```python
from build123d import *

# Parameters (mm, degrees)
F1_DEPTH = 5.08


with BuildPart() as f1:
    # F0 (on Front) → F1 (new body)
    with BuildSketch(Plane.XZ):
        with BuildLine():
            add(Edge.make_bspline(
                [(-88.697367137, -151.6268995181), (-88.8096869402, -151.4451622066), (-75.5090993087, -97.1505766968), (-75.2492718061, -96.7301671852)],
                knots=[0, 0, 0, 0, 1, 1, 1, 1], degree=3))
            add(Edge.make_bspline(
                [(-81.2252771404, -151.7485828201), (-85.2727205926, -151.7823095151), (-88.6351599598, -151.727558088), (-88.697367137, -151.6268995181)],
                knots=[0, 0, 0, 0, 1, 1, 1, 1], degree=3))
            Line((-81.2252771404, -151.7485828201), (-73.8662922876, -151.6872587675))
            Line((-73.8662922876, -151.6872587675), (-70.8277989917, -141.6973681422))
            add(Edge.make_bspline(
                [(-67.6823091824, -131.3943521191), (-67.7411591055, -131.5665717782), (-69.1566280625, -136.202929372), (-70.8277989917, -141.6973681422)],
                knots=[0, 0, 0, 0, 1, 1, 1, 1], degree=3))
            add(Edge.make_bspline(
                [(-64.7710364528, -141.3842427444), (-66.3133869912, -135.7175812475), (-67.6234592594, -131.2221309262), (-67.6823091824, -131.3943521191)],
                knots=[0, 0, 0, 0, 1, 1, 1, 1], degree=3))
            Line((-64.7710364528, -141.3842427444), (-61.9667602367, -151.6872587675))
            Line((-61.9667602367, -151.6872587675), (-54.7617960796, -151.7486058281))
            add(Edge.make_bspline(
                [(-47.327106009, -151.5162830756), (-47.50533383, -151.7441177296), (-49.1720212624, -151.796198692), (-54.7617960796, -151.7486058281)],
                knots=[0, 0, 0, 0, 1, 1, 1, 1], degree=3))
            add(Edge.make_bspline(
                [(-44.3397073984, -141.4129659612), (-45.8564269984, -146.8082708266), (-47.2007536122, -151.3547652154), (-47.327106009, -151.5162830756)],
                knots=[0, 0, 0, 0, 1, 1, 1, 1], degree=3))
            add(Edge.make_bspline(
                [(-41.434975083, -131.8877223747), (-41.5158590234, -131.7313015586), (-42.8229893322, -136.0176626297), (-44.3397073984, -141.4129659612)],
                knots=[0, 0, 0, 0, 1, 1, 1, 1], degree=3))
            add(Edge.make_bspline(
                [(-38.4365004097, -141.6973681422), (-40.0047779231, -136.4584856268), (-41.3540942103, -132.0441447246), (-41.434975083, -131.8877223747)],
                knots=[0, 0, 0, 0, 1, 1, 1, 1], degree=3))
            add(Edge.make_bspline(
                [(-35.35325344, -151.5148749846), (-35.4807623735, -151.3541301939), (-36.8682228963, -146.9362537254), (-38.4365004097, -141.6973681422)],
                knots=[0, 0, 0, 0, 1, 1, 1, 1], degree=3))
            add(Edge.make_bspline(
                [(-21.618593749, -151.747197737), (-32.2466686649, -151.7943779904), (-35.1707783378, -151.744881596), (-35.35325344, -151.5148749846)],
                knots=[0, 0, 0, 0, 1, 1, 1, 1], degree=3))
            Line((-21.618593749, -151.747197737), (-8.1157690404, -151.6872587675))
            Line((-8.1157690404, -151.6872587675), (-8.0551122205, -142.1039337259))
            Line((-8.0551122205, -142.1039337259), (-7.994452333, -132.5206102182))
            Line((-7.994452333, -132.5206102182), (0.0155073543, -132.5206102182))
            Line((0.0155073543, -132.5206102182), (8.0254655077, -132.5206102182))
            Line((8.0254655077, -132.5206102182), (8.0861545387, -141.9877738836))
            Line((8.0861545387, -141.9877738836), (8.1468328327, -151.4549360151))
            Line((8.1468328327, -151.4549360151), (16.8305932312, -151.5710973913))
            add(Edge.make_bspline(
                [(25.602503504, -151.4549360151), (25.5448131854, -151.6069745696), (22.5134799865, -151.6471159016), (16.8305932312, -151.5710973913)],
                knots=[0, 0, 0, 0, 1, 1, 1, 1], degree=3))
            add(Edge.make_bspline(
                [(25.6308616602, -124.1569819276), (25.6637462615, -139.0430796988), (25.6509768084, -151.3271586547), (25.602503504, -151.4549360151)],
                knots=[0, 0, 0, 0, 1, 1, 1, 1], degree=3))
            Line((25.6308616602, -124.1569819276), (25.5710607389, -97.0913505925))
            Line((25.5710607389, -97.0913505925), (16.8589513874, -97.0913505925))
            Line((16.8589513874, -97.0913505925), (8.1468328327, -97.0913505925))
            Line((8.1468328327, -97.0913505925), (8.0863155949, -107.25548194))
            Line((8.0863155949, -107.25548194), (8.0257891539, -117.4196144379))
            Line((8.0257891539, -117.4196144379), (0.0155349639, -117.4196144379))
            Line((0.0155349639, -117.4196144379), (-7.9947238277, -117.4196144379))
            Line((-7.9947238277, -117.4196144379), (-8.055247201, -107.25548194))
            Line((-8.055247201, -107.25548194), (-8.1157690404, -97.0913505925))
            Line((-8.1157690404, -97.0913505925), (-16.0147518261, -97.0913505925))
            Line((-16.0147518261, -97.0913505925), (-23.9137330779, -97.0913505925))
            Line((-23.9137330779, -97.0913505925), (-24.029895988, -118.8869035998))
            Line((-24.029895988, -118.8869035998), (-24.1460573642, -140.682456607))
            Line((-24.1460573642, -140.682456607), (-29.34602871, -119.003064976))
            add(Edge.make_bspline(
                [(-34.7574514629, -96.9138580697), (-34.6411535724, -97.1392555987), (-32.206013487, -107.0794001925), (-29.34602871, -119.003064976)],
                knots=[0, 0, 0, 0, 1, 1, 1, 1], degree=3))
            add(Edge.make_bspline(
                [(-42.3147712321, -96.5653737493), (-35.4953141815, -96.5084380938), (-34.9537513196, -96.5334106193), (-34.7574514629, -96.9138580697)],
                knots=[0, 0, 0, 0, 1, 1, 1, 1], degree=3))
            Line((-42.3147712321, -96.5653737493), (-49.6606411279, -96.6267045125))
            Line((-49.6606411279, -96.6267045125), (-52.2309748268, -106.6762014496))
            add(Edge.make_bspline(
                [(-54.9470536187, -116.3176067958), (-54.8637032182, -116.5509909851), (-53.7009344533, -112.4234481661), (-52.2309748268, -106.6762014496)],
                knots=[0, 0, 0, 0, 1, 1, 1, 1], degree=3))
            add(Edge.make_bspline(
                [(-57.7247095515, -106.5004324194), (-56.2771582062, -111.6754283637), (-55.0272151072, -116.0931558553), (-54.9470536187, -116.3176067958)],
                knots=[0, 0, 0, 0, 1, 1, 1, 1], degree=3))
            add(Edge.make_bspline(
                [(-60.5752196243, -96.8009467685), (-60.4549888956, -96.9606688526), (-59.172257829, -101.3254374338), (-57.7247095515, -106.5004324194)],
                knots=[0, 0, 0, 0, 1, 1, 1, 1], degree=3))
            add(Edge.make_bspline(
                [(-75.2492718061, -96.7301671852), (-75.0293705104, -96.3743622869), (-60.8448337816, -96.4427814387), (-60.5752196243, -96.8009467685)],
                knots=[0, 0, 0, 0, 1, 1, 1, 1], degree=3))
        make_face()
        with BuildLine():
            add(Edge.make_bspline(
                [(-71.5440418374, -137.8059582044), (-69.5220890449, -131.1295757823), (-67.8197054306, -125.5795634317), (-67.7609690139, -125.4725960617)],
                knots=[0, 0, 0, 0, 1, 1, 1, 1], degree=3))
            Line((-71.5440418374, -137.8059582044), (-75.2203236858, -149.9448365905))
            Line((-75.2203236858, -149.9448365905), (-80.8996503329, -149.9448365905))
            add(Edge.make_bspline(
                [(-86.4738924333, -149.5382710068), (-86.5718489025, -149.9172545717), (-86.1936823142, -149.9448365905), (-80.8996503329, -149.9448365905)],
                knots=[0, 0, 0, 0, 1, 1, 1, 1], degree=3))
            add(Edge.make_bspline(
                [(-80.122365283, -123.7504163439), (-83.5579088109, -137.7101251841), (-86.4160974282, -149.3146590921), (-86.4738924333, -149.5382710068)],
                knots=[0, 0, 0, 0, 1, 1, 1, 1], degree=3))
            Line((-80.122365283, -123.7504163439), (-73.8759219124, -98.369127073))
            Line((-73.8759219124, -98.369127073), (-67.9052507966, -98.369127073))
            Line((-67.9052507966, -98.369127073), (-61.9345796809, -98.369127073))
            Line((-61.9345796809, -98.369127073), (-61.695405139, -99.1241769771))
            add(Edge.make_bspline(
                [(-58.3028858485, -111.1468934117), (-60.0372260738, -104.9496764748), (-61.563862132, -99.5394543572), (-61.695405139, -99.1241769771)],
                knots=[0, 0, 0, 0, 1, 1, 1, 1], degree=3))
            add(Edge.make_bspline(
                [(-54.6758104934, -122.835249193), (-54.9802894759, -123.1397297094), (-54.6369790849, -124.2460643938), (-58.3028858485, -111.1468934117)],
                knots=[0, 0, 0, 0, 1, 1, 1, 1], degree=3))
            add(Edge.make_bspline(
                [(-51.3516940574, -110.5413640257), (-53.0491616239, -117.1722030235), (-54.5450114125, -122.704451646), (-54.6758104934, -122.835249193)],
                knots=[0, 0, 0, 0, 1, 1, 1, 1], degree=3))
            Line((-51.3516940574, -110.5413640257), (-48.2653946899, -98.485288641))
            Line((-48.2653946899, -98.485288641), (-42.2075339013, -98.4233886209))
            Line((-42.2075339013, -98.4233886209), (-36.1496731128, -98.3614884092))
            Line((-36.1496731128, -98.3614884092), (-35.7901129215, -99.9334880456))
            add(Edge.make_bspline(
                [(-29.8753911839, -124.6216274325), (-32.9307309547, -111.9077511161), (-35.59235589, -100.7980896958), (-35.7901129215, -99.9334880456)],
                knots=[0, 0, 0, 0, 1, 1, 1, 1], degree=3))
            add(Edge.make_bspline(
                [(-24.1601398086, -148.8458736769), (-24.2481884476, -148.2364156708), (-26.8200498792, -137.3355039405), (-29.8753911839, -124.6216274325)],
                knots=[0, 0, 0, 0, 1, 1, 1, 1], degree=3))
            Line((-24.1601398086, -148.8458736769), (-24.0000530474, -149.9539799791))
            Line((-24.0000530474, -149.9539799791), (-29.0522760681, -149.8913275967))
            Line((-29.0522760681, -149.8913275967), (-34.1044990889, -149.8286752143))
            Line((-34.1044990889, -149.8286752143), (-37.7415461214, -137.7478782833))
            add(Edge.make_bspline(
                [(-41.580826013, -125.6670813523), (-41.4695990909, -125.6670813523), (-39.7419219893, -131.1034402013), (-37.7415461214, -137.7478782833)],
                knots=[0, 0, 0, 0, 1, 1, 1, 1], degree=3))
            add(Edge.make_bspline(
                [(-45.1935198194, -137.7478782833), (-43.3177646111, -131.1034402013), (-41.6920514012, -125.6670813523), (-41.580826013, -125.6670813523)],
                knots=[0, 0, 0, 0, 1, 1, 1, 1], degree=3))
            Line((-45.1935198194, -137.7478782833), (-48.6039853683, -149.8286752143))
            Line((-48.6039853683, -149.8286752143), (-54.5967411191, -149.8286752143))
            Line((-54.5967411191, -149.8286752143), (-60.5894953361, -149.8286752143))
            Line((-60.5894953361, -149.8286752143), (-63.8667827745, -137.8084476726))
            add(Edge.make_bspline(
                [(-67.3991233589, -125.5331654511), (-67.2588434384, -125.6734453716), (-65.6692896386, -131.1973221412), (-63.8667827745, -137.8084476726)],
                knots=[0, 0, 0, 0, 1, 1, 1, 1], degree=3))
            add(Edge.make_bspline(
                [(-67.7609690139, -125.4725960617), (-67.7022341309, -125.3656286918), (-67.5394048133, -125.3928855306), (-67.3991233589, -125.5331654511)],
                knots=[0, 0, 0, 0, 1, 1, 1, 1], degree=3))
        make_face(mode=Mode.SUBTRACT)
        Polygon((-9.7420298412, -131.0105107935), (-9.8027173384, -140.4776729251), (-9.8634033017, -149.9448365905), (-16.1335192445, -149.9448365905), (-22.4036336533, -149.9448365905), (-22.4036336533, -124.38930468), (-22.4036336533, -98.8337731531), (-16.0171937443, -98.8337731531), (-9.6307523015, -98.8337731531), (-9.5702289282, -108.9979050758), (-9.5097070888, -119.162036615), (0.0155349639, -119.162036615), (9.5407739489, -119.162036615), (9.6013003899, -108.9979050758), (9.6618176277, -98.8337731531), (16.8613963734, -98.8337731531), (24.0609674497, -98.8337731531), (24.0609674497, -124.38930468), (24.0609674497, -149.9448365905), (16.8615589634, -149.9448365905), (9.662152011, -149.9448365905), (9.6014629799, -140.4776729251), (9.5407739489, -131.0105107935), (-0.1006279462, -131.0105107935), align=None, mode=Mode.SUBTRACT)
    extrude(amount=F1_DEPTH)


solid = f1.part
```
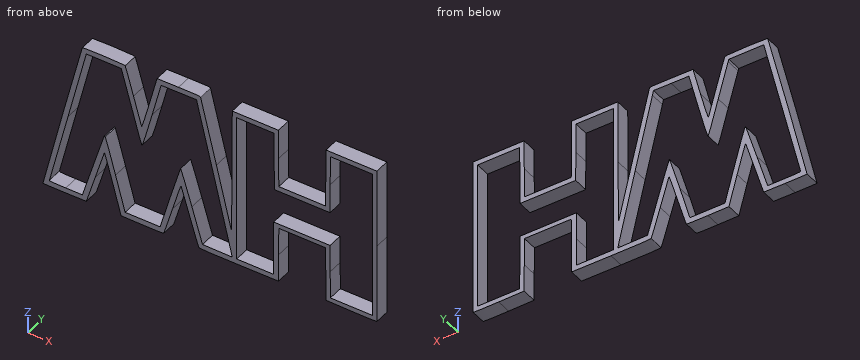
Source: CAD feature listing. Evaluate the final solid. Frame: model axes, mm. Round coordinates to 2 decimals unless told otherwise and drop trailing zeros. Loops run counter-clockwise (first coordinate to the right, second up) from the corner with the lowest first, then second, coordinate; pieces in that order, holes last.
1. Section query A-A on x = 14.5. Output: boundary loops of the cut face in (y, z).
2. Contact query for flat-ended pins moving along their axis: pin 1 (2.5 mm diameter, centred on y = -3.5, z = -115, fed in from -X); pin 2 (1.5 mm diameter, centred on x = 13.5, y = -3, fed in from +Z); pin 3 (1.5 mm diameter, centred on x = -1.5, y = -2, fed in from +Z); pin 4 (10 mm diameter, centred on x = 12.5, z = -128.5, fed in from -Y). Output: stop coordinate, or through.
3. Section query B-B on y = -1.8. Give the number of separate pieces and of enclosed holes in the cut face, and give its area (3 significant figures).
4. Ray query, L1, parallel to Z at x = -12.5, y = -0.6; L2, parallel to Z at x = -2, y = -1.1; L3, parallel to X at y = -4.8, z = -124. Return the intervals inside material, ascending.
Answers below:
1. outline: (-5.08, -151.54) - (0, -151.54) - (0, -149.94) - (-5.08, -149.94) - close; (-5.08, -98.83) - (0, -98.83) - (0, -97.09) - (-5.08, -97.09) - close
2. pin 1: stops at x = -80.14
2. pin 2: stops at z = -97.09
2. pin 3: stops at z = -117.42
2. pin 4: stops at y = -5.08
3. separate pieces: 1
3. enclosed holes: 2
3. area: 1,010 mm2
4. L1: z = -151.71 to -149.94, -98.83 to -97.09
4. L2: z = -132.52 to -131.01, -119.16 to -117.42
4. L3: x = -82.05 to -80.18, -30.02 to -28.15, -24.06 to -22.4, 24.06 to 25.63
